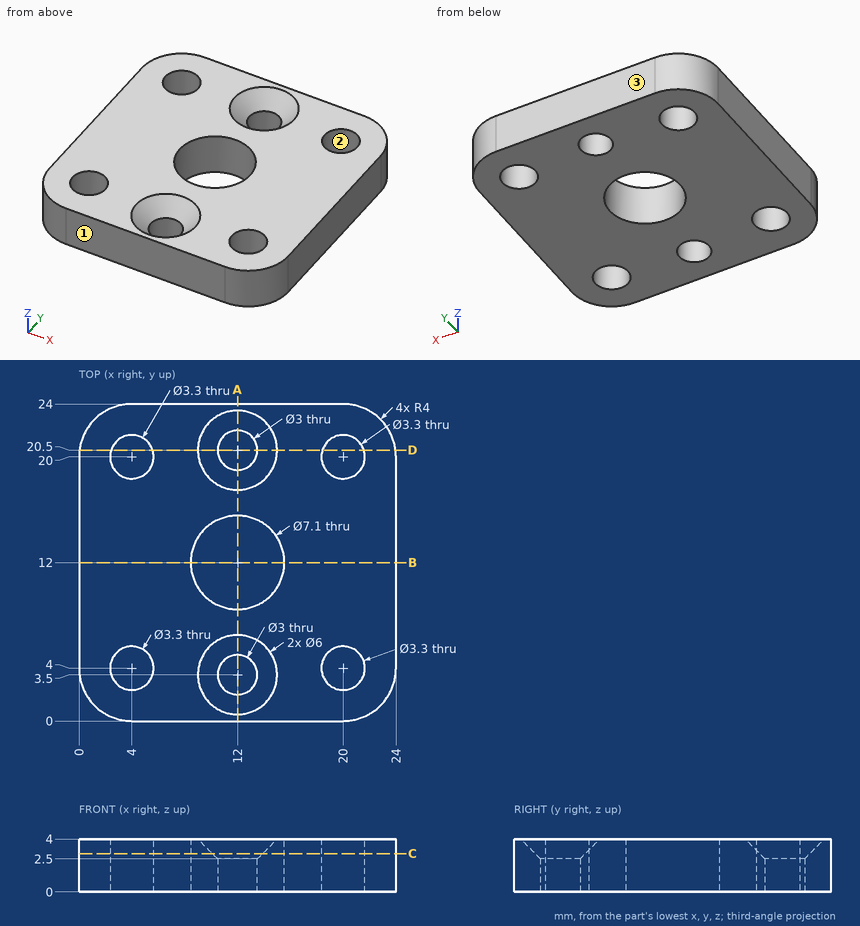
Design review of the part shown in the three views and the two pictorial views. Dimensions are in mm from the part's minimum x, y and z. Coordinates: 2 decimals unless noted, no trailing zeros. Write each loop counter-clockwise with the first axis right and the second up, starting at its lowest first coordinate (ties: lowest second). Pieces come first, ordered by that corner, then holes.
1) Clearance check with a flat-ended pin moving along its axis: pin 1 Ø2.5 at (x, y) = (12, 20.5) entering from -Z. State where the tip first meets the part, or that it passes through.
2) We need section C-C on z = 2.9. State the section outline as (x, y) points.
3) The part is to be moulded in two halves that separate along Y. For the marked faces 1, 2 and 3, say which applies: pulls with the +Y half, pulls with the -Y half, needs draft (parallel to the pull), parting line crosses it, or undercut.
4) We need section D-D on y = 20.5. State the section outline as (x, z) points, then the cut area to 3 significant figures.
5) We need section B-B on y = 12. State the section outline as (x, z) points.
6) We need section A-A on x = 12. State the section outline as (y, z) points, then the cut area to 3 significant figures.
7) To check wall thickness, follow probe 1 along Y at (x, z) = (12, 1.05); probe 2 along Y at (x, z) = (4.25, 2.2); probe 3 along Y at (x, z) = (21, 3.3). State the ranges of each line that lie inside material, in increasing order.
Answer list:
1. pin 1: passes through
2. outline: (0, 4) arc R4 ccw to (4, 0) - (20, 0) arc R4 ccw to (24, 4) - (24, 20) arc R4 ccw to (20, 24) - (4, 24) arc R4 ccw to (0, 20) - close; hole circle Ø3.3 at (4, 4); hole circle Ø3.3 at (4, 20); hole circle Ø7.1 at (12, 12); hole circle Ø3.8 at (12, 3.5); hole circle Ø3.8 at (12, 20.5); hole circle Ø3.3 at (20, 4); hole circle Ø3.3 at (20, 20)
3. face 1: pulls with the -Y half
3. face 2: undercut
3. face 3: pulls with the +Y half
4. outline: (0.03, 0) - (2.43, 0) - (2.43, 4) - (0.03, 4) - close; (5.57, 0) - (10.5, 0) - (10.5, 2.5) - (9, 4) - (5.57, 4) - close; (13.5, 0) - (18.43, 0) - (18.43, 4) - (15, 4) - (13.5, 2.5) - close; (21.57, 0) - (23.97, 0) - (23.97, 4) - (21.57, 4) - close
4. area: 56.3 mm2
5. outline: (0, 0) - (8.45, 0) - (8.45, 4) - (0, 4) - close; (15.55, 0) - (24, 0) - (24, 4) - (15.55, 4) - close
6. outline: (0, 0) - (2, 0) - (2, 2.5) - (0.5, 4) - (0, 4) - close; (5, 0) - (8.45, 0) - (8.45, 4) - (6.5, 4) - (5, 2.5) - close; (15.55, 0) - (19, 0) - (19, 2.5) - (17.5, 4) - (15.55, 4) - close; (22, 0) - (24, 0) - (24, 4) - (23.5, 4) - (22, 2.5) - close
6. area: 39.1 mm2
7. probe 1: y = 0 to 2, 5 to 8.45, 15.55 to 19, 22 to 24
7. probe 2: y = 0 to 2.37, 5.63 to 18.37, 21.63 to 24
7. probe 3: y = 0.13 to 2.69, 5.31 to 18.69, 21.31 to 23.87
